Could you check a few things on this drawing? It's one solid part, dimensions in mm from its lowest x, y, z. Round coordinates to 2 decimals unless told otherwise and drop trailing zeros. Write each loop counter-clockwise with the first axis right and the second up, starting at its lowest first coordinate (ties: lowest second). Pieces come first, ordered by that corner, then holes. Notation, with made-up numbers: (21, 75) - (42, 75) arc R25 ccw to (42, 102) - close; hole circle Ø3 at (78, 17). An arc over 180 degrees is marked (long way). Use one line per item in the form item = value. Start each with the question number.
1. Will these pins go through, and if not, where does the flat tip stop? pin 1 (6 mm diameter, centred on x = 15.5, z = 16.5, fed in from +Y); pin 2 (4 mm diameter, centred on x = 4.5, y = 2.5, fed in from +Z); pin 3 (6 mm diameter, centred on x = 26, y = 2, fed in from +Z).
2. I want a section at B-B, the plane y = 2.5. List the corners of the cut face in (x, z) for me.
3. I want a section at A-A, the plane z = 20. List the corners of the cut face in (x, y) for me (1 decimal).
4. We'd pull the mould along X, two halves only. Please class the marked faces 1, 2 and 3: +X half, -X half, draft (parallel to the pull), parting line (faces both ways), or undercut.
5. If I drill on line 1 along Z through (x, y) = (22, 4.25) (1 decimal); line 2 along X through (y, z) = (4.25, 22); line 3 along Z through (x, y) = (19, 7.5), over which ranges is the centre line in solid material (lowest first)?
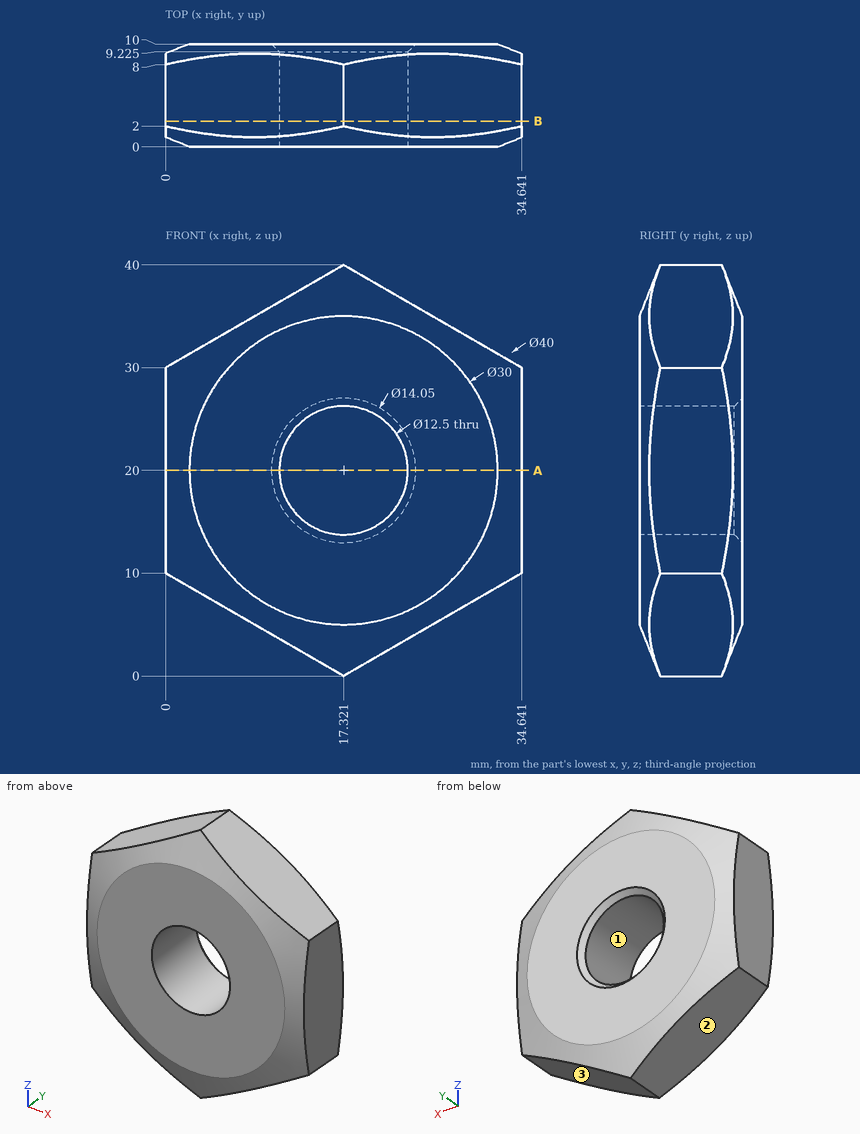
Model answer:
q1.pin_1 = 9.92
q1.pin_2 = 33.75
q1.pin_3 = 36.72
q2.outline = (0, 10) - (17.32, 0) - (34.64, 10) - (34.64, 30) - (17.32, 40) - (0, 30) - close; hole circle Ø12.5 at (17.32, 20)
q3.outline = (0, 0.9) - (2.3, 0) - (11.1, 0) - (11.1, 9.2) - (10.3, 10) - (2.3, 10) - (0, 9.1) - close; (23.6, 0) - (32.3, 0) - (34.6, 0.9) - (34.6, 9.1) - (32.3, 10) - (24.3, 10) - (23.6, 9.2) - close
q4.face_1 = undercut
q4.face_2 = -X half
q4.face_3 = +X half
q5.line_1 = 2.7 to 15.9, 24.1 to 37.3
q5.line_2 = 0 to 11.4, 23.24 to 34.64
q5.line_3 = 0.97 to 13.98, 26.02 to 39.03
